from build123d import *

# Parameters (mm, degrees)
F0_W     = 152.4
F0_H     = 50.8
F1_DEPTH = 4.7625
F2_W     = 19.05
F2_H     = 4.7625
F2_W_2   = 12.7
F3_DEPTH = 25.4
F4_W     = 4.7625
F4_H     = 12.7
F5_DEPTH = 25.4


with BuildPart() as f1:
    # F0 (on Top) → F1 (new body)
    with BuildSketch(Plane.XY):
        Rectangle(F0_W, F0_H)
    extrude(amount=F1_DEPTH)

    # F2 (on face) → F3 (cut)
    with BuildSketch(Plane.XY.offset(4.7625)):
        with Locations((-66.675, -23.01875)):
            Rectangle(F2_W, F2_H)
        with Locations((-38.1, -23.01875)):
            Rectangle(F2_W_2, F2_H)
        with Locations((-12.7, -23.01875)):
            Rectangle(F2_W_2, F2_H)
        with Locations((12.7, -23.01875)):
            Rectangle(F2_W_2, F2_H)
        with Locations((66.675, -23.01875)):
            Rectangle(F2_W, F2_H)
        with Locations((38.1, -23.01875)):
            Rectangle(F2_W_2, F2_H)
    extrude(amount=-F3_DEPTH, mode=Mode.SUBTRACT)

    # F4 (on face) → F5 (cut)
    with BuildSketch(Plane.XY.offset(4.7625)):
        with Locations((-73.81875, 19.05)):
            Rectangle(F4_W, F4_H)
        with Locations((-73.81875, -14.2875)):
            Rectangle(F4_W, F4_H)
        with Locations((73.81875, 19.05)):
            Rectangle(F4_W, F4_H)
        with Locations((73.81875, -14.2875)):
            Rectangle(F4_W, F4_H)
    extrude(amount=-F5_DEPTH, mode=Mode.SUBTRACT)


solid = f1.part
Read the model definition and answer for the solid it produces. Units are mm, in the model's axes. A direction names the side the tool comes from. Coordinates: 2 decimals unless noted, no trailing zeros. Loops run counter-clockwise (first coordinate to the right, second up) from the corner with the lowest first, then second, coordinate; pieces in that order, holes last. Notation, with made-up numbers: (-11, -34.5) -> (34, -34.5) arc R18 ccw to (34, -9.5) -> close; hole circle Ø5 at (-17.75, 17). An arc over 180 degrees is marked (long way). Write item = value, one per line. Start each with the question number.
1) The mould has two halves that part along X. Classify faces 5 (the face through (71.438, -14, 2)), 6 (the face through (0, -25.4, 2)), 7 (the face through (-76.2, 2, 2)), 8 (the face through (31.75, -23, 2)): pulls with the +X half, pulls with the -X half, needs draft (parallel to the pull), parting line crosses it, or undercut.
2) The part is cut by section B-B, the plane y = 17.5. Determine the outline of the cut face in (x, z), plus the area to 3 significant figures.
3) For faces 1 (the face through (-38, -20.638, 2)), 2 (the face through (57.15, -23, 2)), 3 (the face through (71.438, 19, 2)), 4 (the face through (-71.438, 19, 2)), determine the directions among +Z, -Z, +X, -X, +Y, -Y from which every point of the face is accessible in a straight line to the end or side of a thin tool.
4) Given P1, Ø1.4, axis at y = 19, z = 2, coming from the -X side; P2, Ø1.4, axis at y = -23.5, z = 3.5, coming from the -X side; P3, Ø2.5, axis at x = 74, z = 2, coming from the -Y side, each flat-ended and moving along its own axis, determine where each tip first touches the part or whether it passes through.
5) Find the intervals of material crossed by L1, parallel to X at y = -22, z = 1; L2, parallel to Y at x = 8.5, z = 3.6; L3, parallel to X at y = 23.5, z = 0.6, in increasing order. Write a range as from..to.
6) The part is cut by section C-C, the plane x = -16. Determine the outline of the cut face in (y, z), plus the area to 3 significant figures.
Result:
q1.face_5 = pulls with the +X half
q1.face_6 = needs draft
q1.face_7 = pulls with the -X half
q1.face_8 = undercut
q2.outline = (-71.44, 0) -> (71.44, 0) -> (71.44, 4.76) -> (-71.44, 4.76) -> close
q2.area = 680 mm²
q3.face_1 = +Z, -Z, -Y
q3.face_2 = +Z, -Z, +X, -Y
q3.face_3 = +Z, -Z, +X, +Y
q3.face_4 = +Z, -Z, -X, +Y
q4.P1 = -71.44
q4.P2 = -57.15
q4.P3 = -7.94
q5.L1 = -57.15..-44.45, -31.75..-19.05, -6.35..6.35, 19.05..31.75, 44.45..57.15
q5.L2 = -20.64..25.4
q5.L3 = -71.44..71.44
q6.outline = (-20.64, 0) -> (25.4, 0) -> (25.4, 4.76) -> (-20.64, 4.76) -> close
q6.area = 219 mm²
